```python
from build123d import *

# Parameters (mm, degrees)
BOSS_EXTRU_1_DEPTH      = 1.6
ESQUISSE2_R             = 0.5
ENL_V_MAT_EXTRU_1_DEPTH = 2.6
BOSS_EXTRU_2_DEPTH      = 4.5
ESQUISSE5_W             = 62
ESQUISSE5_H             = 16
ENL_V_MAT_EXTRU_2_DEPTH = 0.2
ESQUISSE6_W             = 2.78
ESQUISSE6_H             = 4.89
ENL_V_MAT_EXTRU_3_DEPTH = 0.1


with BuildPart() as part:
    # Esquisse1 → Boss.-Extru.1 (new body)
    with BuildSketch(Plane(origin=(0, 0, 0), x_dir=(1, 0, 0), z_dir=(0, 1, 0))):
        with BuildLine():
            Line((-41, -13.25), (-42.5, -13.25))
            Line((-42.5, -13.25), (-42.5, -15))
            Line((-42.5, -15), (42.5, -15))
            Line((42.5, -15), (42.5, -13.25))
            Line((42.5, -13.25), (41, -13.25))
            ThreePointArc((41, -13.25), (39.75, -12), (41, -10.75))
            Line((41, -10.75), (42.5, -10.75))
            Line((42.5, -10.75), (42.5, 10.75))
            Line((42.5, 10.75), (41, 10.75))
            ThreePointArc((41, 10.75), (39.75, 12), (41, 13.25))
            Line((41, 13.25), (42.5, 13.25))
            Line((42.5, 13.25), (42.5, 15))
            Line((42.5, 15), (-42.5, 15))
            Line((-42.5, 15), (-42.5, 13.25))
            Line((-42.5, 13.25), (-41, 13.25))
            ThreePointArc((-41, 13.25), (-39.75, 12), (-41, 10.75))
            Line((-41, 10.75), (-42.5, 10.75))
            Line((-42.5, 10.75), (-42.5, -10.75))
            Line((-42.5, -10.75), (-41, -10.75))
            ThreePointArc((-41, -10.75), (-39.75, -12), (-41, -13.25))
        make_face()
    extrude(amount=BOSS_EXTRU_1_DEPTH)

    # Esquisse2 → Enlèv. mat.-Extru.1 (cut, through all)
    with BuildSketch(Plane.XZ):
        with Locations((-41, 7.62)):
            Circle(ESQUISSE2_R)
        with Locations((-38.46, 7.62)):
            Circle(ESQUISSE2_R)
        with Locations((-38.46, 5.08)):
            Circle(ESQUISSE2_R)
        with Locations((-38.46, 2.54)):
            Circle(ESQUISSE2_R)
        with Locations((-38.46, 0)):
            Circle(ESQUISSE2_R)
        with Locations((-38.46, -2.54)):
            Circle(ESQUISSE2_R)
        with Locations((-38.46, -5.08)):
            Circle(ESQUISSE2_R)
        with Locations((-38.46, -7.62)):
            Circle(ESQUISSE2_R)
        with Locations((-41, 5.08)):
            Circle(ESQUISSE2_R)
        with Locations((-41, 2.54)):
            Circle(ESQUISSE2_R)
        with Locations((-41, 0)):
            Circle(ESQUISSE2_R)
        with Locations((-41, -2.54)):
            Circle(ESQUISSE2_R)
        with Locations((-41, -5.08)):
            Circle(ESQUISSE2_R)
        with Locations((-41, -7.62)):
            Circle(ESQUISSE2_R)
    extrude(amount=-ENL_V_MAT_EXTRU_1_DEPTH, mode=Mode.SUBTRACT)

    # Esquisse3 → Boss.-Extru.2 (add)
    with BuildSketch(Plane.XZ):
        Polygon((-34.75, 13.3), (-34.75, 11.95), (-36.25, 11.95), (-36.25, -11.95), (-34.75, -11.95), (-34.75, -13.3), (34.75, -13.3), (34.75, -11.95), (36.25, -11.95), (36.25, 11.95), (34.75, 11.95), (34.75, 13.3), align=None)
    extrude(amount=BOSS_EXTRU_2_DEPTH)

    # Esquisse5 → Enlèv. mat.-Extru.2 (cut)
    with BuildSketch(Plane.XZ.offset(4.5)):
        Rectangle(ESQUISSE5_W, ESQUISSE5_H)
    extrude(amount=-ENL_V_MAT_EXTRU_2_DEPTH, mode=Mode.SUBTRACT)

    # Esquisse6 → Enlèv. mat.-Extru.3 (cut)
    with BuildSketch(Plane.XZ.offset(4.3)):
        with Locations((26.475, -3.045)):
            Rectangle(ESQUISSE6_W, ESQUISSE6_H)
        with Locations((22.995, -3.045)):
            Rectangle(ESQUISSE6_W, ESQUISSE6_H)
        with Locations((19.515, -3.045)):
            Rectangle(ESQUISSE6_W, ESQUISSE6_H)
        with Locations((16.035, -3.045)):
            Rectangle(ESQUISSE6_W, ESQUISSE6_H)
        with Locations((12.555, -3.045)):
            Rectangle(ESQUISSE6_W, ESQUISSE6_H)
        with Locations((9.075, -3.045)):
            Rectangle(ESQUISSE6_W, ESQUISSE6_H)
        with Locations((5.595, -3.045)):
            Rectangle(ESQUISSE6_W, ESQUISSE6_H)
        with Locations((2.115, -3.045)):
            Rectangle(ESQUISSE6_W, ESQUISSE6_H)
        with Locations((-1.365, -3.045)):
            Rectangle(ESQUISSE6_W, ESQUISSE6_H)
        with Locations((-4.845, -3.045)):
            Rectangle(ESQUISSE6_W, ESQUISSE6_H)
        with Locations((-8.325, -3.045)):
            Rectangle(ESQUISSE6_W, ESQUISSE6_H)
        with Locations((-11.805, -3.045)):
            Rectangle(ESQUISSE6_W, ESQUISSE6_H)
        with Locations((-15.285, -3.045)):
            Rectangle(ESQUISSE6_W, ESQUISSE6_H)
        with Locations((-18.765, -3.045)):
            Rectangle(ESQUISSE6_W, ESQUISSE6_H)
        with Locations((-22.245, -3.045)):
            Rectangle(ESQUISSE6_W, ESQUISSE6_H)
        with Locations((-25.725, -3.045)):
            Rectangle(ESQUISSE6_W, ESQUISSE6_H)
        with Locations((26.475, 2.955)):
            Rectangle(ESQUISSE6_W, ESQUISSE6_H)
        with Locations((22.995, 2.955)):
            Rectangle(ESQUISSE6_W, ESQUISSE6_H)
        with Locations((19.515, 2.955)):
            Rectangle(ESQUISSE6_W, ESQUISSE6_H)
        with Locations((16.035, 2.955)):
            Rectangle(ESQUISSE6_W, ESQUISSE6_H)
        with Locations((12.555, 2.955)):
            Rectangle(ESQUISSE6_W, ESQUISSE6_H)
        with Locations((9.075, 2.955)):
            Rectangle(ESQUISSE6_W, ESQUISSE6_H)
        with Locations((5.595, 2.955)):
            Rectangle(ESQUISSE6_W, ESQUISSE6_H)
        with Locations((2.115, 2.955)):
            Rectangle(ESQUISSE6_W, ESQUISSE6_H)
        with Locations((-1.365, 2.955)):
            Rectangle(ESQUISSE6_W, ESQUISSE6_H)
        with Locations((-4.845, 2.955)):
            Rectangle(ESQUISSE6_W, ESQUISSE6_H)
        with Locations((-8.325, 2.955)):
            Rectangle(ESQUISSE6_W, ESQUISSE6_H)
        with Locations((-11.805, 2.955)):
            Rectangle(ESQUISSE6_W, ESQUISSE6_H)
        with Locations((-15.285, 2.955)):
            Rectangle(ESQUISSE6_W, ESQUISSE6_H)
        with Locations((-18.765, 2.955)):
            Rectangle(ESQUISSE6_W, ESQUISSE6_H)
        with Locations((-22.245, 2.955)):
            Rectangle(ESQUISSE6_W, ESQUISSE6_H)
        with Locations((-25.725, 2.955)):
            Rectangle(ESQUISSE6_W, ESQUISSE6_H)
    extrude(amount=-ENL_V_MAT_EXTRU_3_DEPTH, mode=Mode.SUBTRACT)


solid = part.part
```
Source: CAD feature listing. Evaluate the final solid. Frame: model axes, mm. A direction names the side the tool comes from. Coordinates: 2 decimals unless noted, no trailing zeros. Write each loop counter-clockwise with the first axis right and the second up, starting at its lowest first coordinate (ties: lowest second). Pieces come first, ordered by that corner, then holes. Notation, with made-up numbers: (86.5, 27.5) - (92.5, 27.5) arc R14 ccw to (92.5, 46.5) - close; hole circle Ø2 at (-4.75, 5). An arc over 180 degrees is marked (long way). Answer as a JSON object with one key per item and string values.
Q1. Material intervals for line 1 (X direction, y = 0.75, z = 2.75); line 2 (Y direction, x = 22, z = 5.5); line 3 (Z direction, x = 14, y = -1.75), sorted ascending. Write a range as [from, to].
Ans:
{"line 1": "x = [-42.5, -41.45], [-40.55, -38.91], [-38.01, 42.5]", "line 2": "y = [-4.3, 1.6]", "line 3": "z = [-13.3, 13.3]"}
Q2. Section query B-B, the plane y = -1. Output: boundary loops of the cut face in (x, z).
Ans:
{"outline": "(-36.25, -11.95) - (-34.75, -11.95) - (-34.75, -13.3) - (34.75, -13.3) - (34.75, -11.95) - (36.25, -11.95) - (36.25, 11.95) - (34.75, 11.95) - (34.75, 13.3) - (-34.75, 13.3) - (-34.75, 11.95) - (-36.25, 11.95) - close"}
Q3. First-contact query: pin 1 Ø0.8 at (x, z) = (-15, -3) entering from -Y; pin 2 Ø2 at (x, z) = (-11, -2.5) entering from -Y. Flat tips, straight axial feed; report the tip coordinate or a pass-through.
Ans:
{"pin 1": "stops at y = -4.2", "pin 2": "stops at y = -4.3"}
Q4. Set-up query: faces 4 (the flat face through (0, -2, 13.3)), 5 (the flat face through (-42, 1, 13.25)), 6 (the flat face through (42, 1, -13.25)), 7 (the flat face through (6, -4.2, 3)). Return all of +Z, -Z, +X, -X, +Y, -Y with unobstructed straight access to the full face (end or side cutting, diameter ignored); none if empty.
Ans:
{"face 4": "+Z, +X, -X, -Y", "face 5": "-X, +Y, -Y", "face 6": "+X, +Y, -Y", "face 7": "-Y"}
Q5. Draft query along X for faces 1 (the flat face through (13, -4.2, -3)), 2 (the flat face through (42, 1, -10.75)), 3 (the flat face through (-42.5, 1, 14)). Return one class per face: released by +X, released by -X, zero draft, split by the parting line, or undercut.
Ans:
{"face 1": "undercut", "face 2": "zero draft", "face 3": "released by -X"}
Q6. Section query A-A, the plane z = 9.75. Output: boundary loops of the cut face in (x, y).
Ans:
{"outline": "(-42.5, 0) - (-36.25, 0) - (-36.25, -4.5) - (36.25, -4.5) - (36.25, 0) - (42.5, 0) - (42.5, 1.6) - (-42.5, 1.6) - close"}
